```python
from build123d import *

# Parameters (mm, degrees)
BOSS_EXTRUDE1_DEPTH = 69
SKETCH2_W           = 69
SKETCH2_H           = 2
BOSS_EXTRUDE2_DEPTH = 3
SKETCH3_W           = 5
SKETCH3_H           = 7
BOSS_EXTRUDE4_DEPTH = 13
SKETCH5_R           = 1.5
BOSS_EXTRUDE5_DEPTH = 3
SKETCH8_W           = 10
SKETCH8_H           = 14
CUT_EXTRUDE1_DEPTH  = 71.372224634
CUT_EXTRUDE2_DEPTH  = 3


with BuildPart() as part:
    # Sketch1 → Boss-Extrude1 (new body)
    with BuildSketch(Plane.XY):
        Polygon((2.5, 1), (2.5, 8), (-7.5, 8), (-7.5, 10), (7.5, 10), (7.5, 1), align=None)
    extrude(amount=-BOSS_EXTRUDE1_DEPTH)

    # Sketch2 → Boss-Extrude2 (add)
    with BuildSketch(Plane.ZY.offset(7.5)):
        with Locations((-34.5, 9)):
            Rectangle(SKETCH2_W, SKETCH2_H)
    extrude(amount=BOSS_EXTRUDE2_DEPTH)

    # Sketch3 → Boss-Extrude4 (add)
    with BuildSketch(Plane.ZY.offset(-2.5)):
        with Locations((-34.5, 4.5)):
            Rectangle(SKETCH3_W, SKETCH3_H)
    extrude(amount=BOSS_EXTRUDE4_DEPTH)

    # Sketch5 → Boss-Extrude5 (add)
    with BuildSketch(Plane.XY.offset(-32)):
        with Locations(Location((-2.5, 4.5, 0), (0, 0, 180))):
            Circle(SKETCH5_R)
    boss_extrude5 = extrude(amount=BOSS_EXTRUDE5_DEPTH)

    # Sketch8 → Cut-Extrude1 (cut, through all)
    with BuildSketch(Plane(origin=(0, 10, 0), x_dir=(1, 0, 0), z_dir=(0, 1, 0))):
        with Locations((-2.5, 10)):
            Rectangle(SKETCH8_W, SKETCH8_H)
    cut_extrude1 = extrude(amount=-CUT_EXTRUDE1_DEPTH, mode=Mode.SUBTRACT)

    # Mirror1: Boss-Extrude5, Cut-Extrude1 across plane
    add(boss_extrude5.mirror(Plane.XY.offset(-34.5)))
    add(cut_extrude1.mirror(Plane.XY.offset(-34.5)), mode=Mode.SUBTRACT)

    # Sketch9 → Cut-Extrude2 (cut)
    with BuildSketch(Plane.XZ.offset(-1)):
        with BuildLine():
            Line((6.6, -24.5), (6.6, -44.5))
            ThreePointArc((6.6, -44.5), (5, -46.1), (3.4, -44.5))
            Line((3.4, -44.5), (3.4, -24.5))
            ThreePointArc((3.4, -24.5), (5, -22.9), (6.6, -24.5))
        make_face()
    extrude(amount=-CUT_EXTRUDE2_DEPTH, mode=Mode.SUBTRACT)


solid = part.part
```
CAD build for the part. Positions are in the model's coordinates, mm. A direction names the side the tool comes from. Give positions to 0.01 mm unless a question says otherwise; leave off trailing zeros. Order: outer loops, then holes, each group sorted by start corner. A loop starts at its lowest first (then second) coordinate and runs counter-clockwise, first axis right, second up.
(1) Tool access for faces 5 (the flat face through (-2, 4, -40)), 6 (the cylindrical face through (-2.305, 3.013, -38.479)), 7 (the flat face through (-3, 9, -52)), 8 (the cylindrical face through (5, 2.5, -22.9)): list every direction of +Z, -Z, +X, -X, +Y, -Y with a clear straight run to the whole face (end or side of a thin tool).
(2) Saw through at C-C, the plane y = 8.75. Give the cut face in (x, z).
(3) Saw through at A-A, the plane x = 1.5. Give the cut face in (y, z).
(4) Mould opens along X. For faces 1 (the flat face through (-10.5, 8, -35)), 2 (the flat face through (-2, 4, -29)), 3 (the flat face through (-7.5, 9, -59)), 4 (the cylindrical face through (-2.305, 3.013, -30.521)) say: released by +X, released by -X, zero draft, split by the parting line, or undercut.
(5) Drill centre lines: L1, parallel to Z at x = -5, y = 9.25; L2, parallel to X at y = 8.75, z = -63; L3, parallel to Y at x = 1.75, z = -25. Where is each one in solid material? Low to high.
(6) Saw through at D-D, the plane x = -8.75. Give the cut face in (y, z).
(7) Flat gauge pins, fed straight in: pin 1 (5 mm diameter, centred on x = -5.5, z = -19.5, fed in from -Y); pin 2 (2.5 mm diameter, centred on x = -2, y = 5, fed in from -Z); pin 3 (2.5 mm diameter, centred on x = -2, y = 4, fed in from +Z). Where does each tip first touch, or does it go through?
(8) Saw through at B-B, the plane z = -53.5. Give the cut face in (x, y).
Results found:
1. face 5: -Z, -X, -Y
1. face 6: -Z
1. face 7: +Y, -Y
1. face 8: -Y
2. outline: (-10.5, -69) - (7.5, -69) - (7.5, 0) - (-10.5, 0) - close; hole (-7.5, -66) - (2.5, -66) - (2.5, -52) - (-7.5, -52) - close; hole (-7.5, -17) - (2.5, -17) - (2.5, -3) - (-7.5, -3) - close
3. outline: (1, -37) - (8, -37) - (8, -52) - (10, -52) - (10, -17) - (8, -17) - (8, -32) - (1, -32) - close; (8, -69) - (10, -69) - (10, -66) - (8, -66) - close; (8, -3) - (10, -3) - (10, 0) - (8, 0) - close
4. face 1: released by -X
4. face 2: zero draft
4. face 3: undercut
4. face 4: undercut
5. L1: z = -69 to -66, -52 to -17, -3 to 0
5. L2: x = -10.5 to -7.5, 2.5 to 7.5
5. L3: y = 8 to 10
6. outline: (1, -37) - (8, -37) - (8, -69) - (10, -69) - (10, 0) - (8, 0) - (8, -32) - (1, -32) - close
7. pin 1: stops at y = 8
7. pin 2: stops at z = -40
7. pin 3: stops at z = -29
8. outline: (-10.5, 8) - (-7.5, 8) - (-7.5, 10) - (-10.5, 10) - close; (2.5, 1) - (7.5, 1) - (7.5, 10) - (2.5, 10) - close
